Job drawing, mm, ordinate dimensions from the low corner. One solid piece. A direction names the side the tool comes from. Give positions to 0.01 mm unless a question says otherwise; leave off trailing zeros. Write each loop counter-clockwise with the first axis right and the second up, starting at its lowest first coordinate (ties: lowest second). Pieces come first, ordered by that corner, then holes. Notation, with made-up numbers: (27.5, -12) -> (84.5, -12) arc R11 ccw to (84.5, 9) -> close; hole circle Ø4 at (32, 33.25). An arc over 180 degrees is marked (long way). One line per question, with ' | ' between items. Start each with the question number.
(1) Band-saw the part on A-A, the plane x = 96. Give the cut face in (y, z), and give its area (3 significant figures).
(2) Pull direction X, two halves, no side cores. Call the marked faces 4, 5 and 6: released by +X, released by -X, zero draft, split by the parting line, or undercut.
(3) Band-saw the part on B-B, the plane y = 28.5. Give the cut face in (x, z), and give its area (3 significant figures).
(4) Pin check, flat tips, straight feed: P1, Ø16.5, axis at x = 102, y = 36.5, coming from the +Z side; P2, Ø5, axis at x = 87.5, y = 34, coming from the -Z side; P3, Ø2, axis at x = 87.16, y = 37.34, coming from the +Z side; P4, Ø4, axis at x = 31, z = 20, coming from the +Y side. Stop position of each tip, or through.
(5) Band-saw the part on D-D, the plane z = 47. Give the cut face in (x, y).
(6) Drill centre lines: probe 1 along Z at (x, y) = (127, 1.05); probe 2 along Z at (x, y) = (127, 5.4); probe 3 along X at (y, z) = (20, 19). Where is each one in solid material? Low to high. Write a range as from..to.
(7) Band-saw the part on C-C, the plane x = 127. Give the cut face in (y, z), and give its area (3 significant figures).
(8) Tool access for the marked faces 1, 2 and 3: list every direction of +Z, -Z, +X, -X, +Y, -Y with a clear straight run to the whole face (end or side of a thin tool).
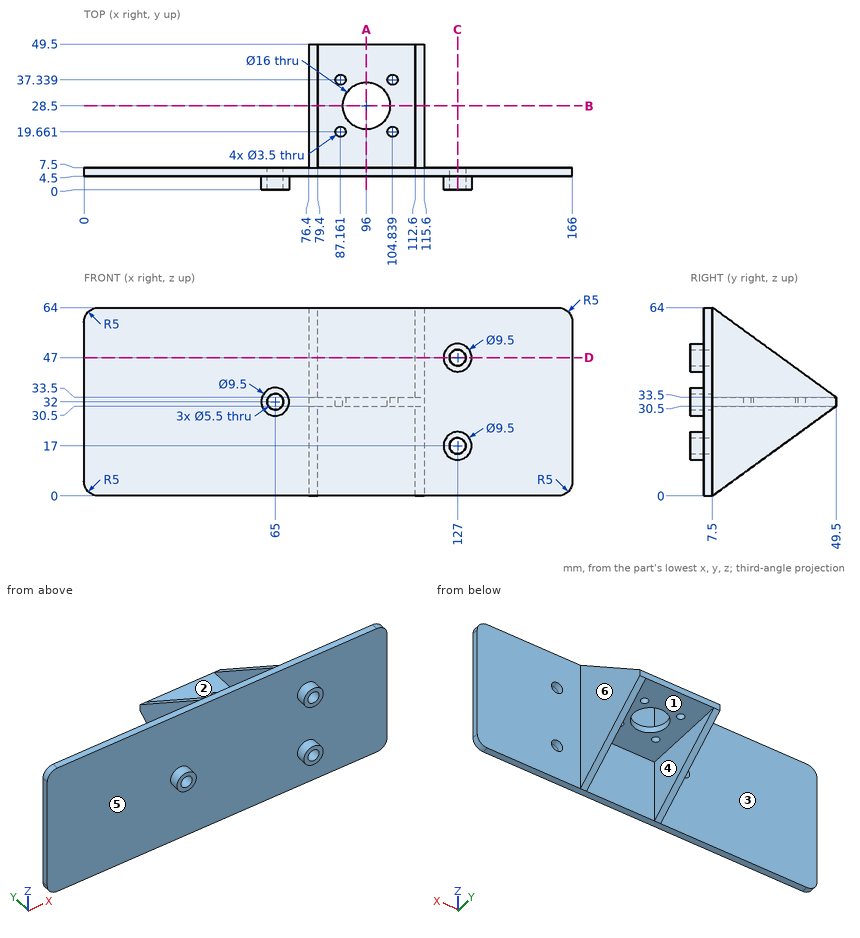
Results:
1) outline: (4.5, 0) -> (7.5, 0) -> (7.5, 30.5) -> (20.5, 30.5) -> (20.5, 33.5) -> (7.5, 33.5) -> (7.5, 64) -> (4.5, 64) -> close; (36.5, 30.5) -> (49.5, 30.5) -> (49.5, 33.5) -> (36.5, 33.5) -> close | area: 270 mm²
2) face 4: undercut | face 5: zero draft | face 6: released by +X
3) outline: (76.4, 15.25) -> (79.4, 15.25) -> (79.4, 30.5) -> (88, 30.5) -> (88, 33.5) -> (79.4, 33.5) -> (79.4, 48.75) -> (76.4, 48.75) -> close; (104, 30.5) -> (112.6, 30.5) -> (112.6, 15.25) -> (115.6, 15.25) -> (115.6, 48.75) -> (112.6, 48.75) -> (112.6, 33.5) -> (104, 33.5) -> close | area: 253 mm²
4) P1: stops at z = 33.5 | P2: stops at z = 30.5 | P3: passes through | P4: stops at y = 7.5
5) outline: (0, 4.5) -> (122.25, 4.5) -> (122.25, 0) -> (124.25, 0) -> (124.25, 7.5) -> (115.6, 7.5) -> (115.6, 30.91) -> (112.6, 30.91) -> (112.6, 7.5) -> (79.4, 7.5) -> (79.4, 30.91) -> (76.4, 30.91) -> (76.4, 7.5) -> (0, 7.5) -> close; (129.75, 0) -> (131.75, 0) -> (131.75, 4.5) -> (166, 4.5) -> (166, 7.5) -> (129.75, 7.5) -> close
6) probe 1: z = 12.25..14.25, 19.75..21.75, 42.25..44.25, 49.75..51.75 | probe 2: z = 0..14.25, 19.75..44.25, 49.75..64 | probe 3: x = 76.4..79.4, 112.6..115.6
7) outline: (0, 12.25) -> (4.5, 12.25) -> (4.5, 0) -> (7.5, 0) -> (7.5, 14.25) -> (0, 14.25) -> close; (0, 19.75) -> (7.5, 19.75) -> (7.5, 44.25) -> (0, 44.25) -> (0, 42.25) -> (4.5, 42.25) -> (4.5, 21.75) -> (0, 21.75) -> close; (0, 49.75) -> (7.5, 49.75) -> (7.5, 64) -> (4.5, 64) -> (4.5, 51.75) -> (0, 51.75) -> close | area: 195 mm²
8) face 1: -Z, +Y | face 2: +Z, +Y | face 3: +Z, -Z, -X, +Y
